```python
from build123d import *

# Parameters (mm, degrees)
F1_DEPTH = 150
F3_DEPTH = 200
F5_DEPTH = 100
F6_R     = 5
F7_R     = 5
F8_R     = 5
F9_R     = 5
F10_R    = 5
F11_R    = 5
F12_R    = 5


with BuildPart() as f1:
    # F0 (on Front) → F1 (new body)
    with BuildSketch(Plane.XZ):
        Polygon((2.699633, 10.554306), (13.111226, -10.555131), (91.699633, 13.444814), (91.699633, 51.205629), (2.699633, 51.205629), (-87.100367, 51.205629), (-87.100367, 12.852651), (-8.070518, -11.282105), align=None)
    extrude(amount=F1_DEPTH)

    # F2 (on face) → F3 (cut)
    with BuildSketch(Plane(origin=(0, 0, 0), x_dir=(-1, 0, 0), z_dir=(0, 1, 0))):
        Polygon((10.674811, -5.258827), (82.100367, 16.55367), (82.100367, 46.205629), (-86.699632, 46.205629), (-86.699632, 17.145834), (-15.715518, -4.531853), (-2.699633, 21.857769), align=None)
    extrude(amount=-F3_DEPTH, mode=Mode.SUBTRACT)

    # F4 (on face) → F5 (intersect)
    with BuildSketch(Plane.XY.offset(51.205629)):
        with BuildLine():
            Line((105.917034, -74.399856), (110.162811, -71.75914))
            ThreePointArc((110.162811, -71.75914), (-2.511346, -9.56452), (-114.475567, -73.028285))
            Line((-114.475567, -73.028285), (-110.200224, -75.620859))
            ThreePointArc((-110.200224, -75.620859), (-2.483098, -14.564441), (105.917034, -74.399856))
        make_face()
    extrude(amount=-F5_DEPTH, mode=Mode.INTERSECT)

    # F6
    f6_edges = [f1.edges().sort_by_distance(p)[0] for p in [
        (2.699633, -12.139598, 21.857769),
    ]]
    fillet(f6_edges, radius=F6_R)

    # F7
    f7_edges = [f1.edges().sort_by_distance(p)[0] for p in [
        (-8.070518, -12.216219, -11.282105),
    ]]
    fillet(f7_edges, radius=F7_R)

    # F8
    f8_edges = [f1.edges().sort_by_distance(p)[0] for p in [
        (13.111226, -12.92147, -10.555131),
    ]]
    fillet(f8_edges, radius=F8_R)

    # F9
    f9_edges = [f1.edges().sort_by_distance(p)[0] for p in [
        (-87.100367, -44.240648, 51.205629),
    ]]
    fillet(f9_edges, radius=F9_R)

    # F10
    f10_edges = [f1.edges().sort_by_distance(p)[0] for p in [
        (-87.100367, -44.240648, 12.852651),
    ]]
    fillet(f10_edges, radius=F10_R)

    # F11
    f11_edges = [f1.edges().sort_by_distance(p)[0] for p in [
        (91.699633, -52.049978, 51.205629),
    ]]
    fillet(f11_edges, radius=F11_R)

    # F12
    f12_edges = [f1.edges().sort_by_distance(p)[0] for p in [
        (91.699633, -52.049978, 13.444814),
    ]]
    fillet(f12_edges, radius=F12_R)


solid = f1.part
```
Can you work these out from the model? Positions are in its coordinate system, mm. A direction names the side the tool comes from. Give positions to 0.01 mm unless a question says otherwise; leave off trailing zeros. Order: outer loops, then holes, each group sorted by start corner. A loop starts at its lowest first (then second) coordinate and runs counter-clockwise, first axis right, second up. Notation, with made-up numbers: M 3,-10 L 24,-10 A7 ccw 24,-2 Z; hole C -13.5,-37.75 d4. An arc over 180 degrees is marked long. One line per item, written item: value.
1) I want a section at A-A, the plane z = 24.5. List the corners of the cut face in (x, y) for me.
Answer sheet:
outline: M -87.1,-47.57 A126.81 cw -82.1,-43.25 L -82.1,-36.87 A131.81 ccw -87.1,-40.91 Z; M 86.7,-50.52 A126.81 cw 91.7,-55.67 L 91.7,-48.43 A131.81 ccw 86.7,-43.66 Z
2) I want a section at D-D, the plane z = -2.5. List the corners of the cut face in (x, y) for me.
Answer sheet:
outline: M -36.83,-19.51 A126.81 cw -19.71,-15.84 L -19.71,-10.79 A131.81 ccw -36.83,-14.31 Z; M -9.31,-14.79 A126.81 cw -3.74,-14.58 L -3.74,-9.58 A131.81 ccw -9.31,-9.78 Z; M 9.14,-15.03 A126.81 cw 14.71,-15.64 L 14.71,-10.6 A131.81 ccw 9.14,-10.01 Z; M 22.37,-16.88 A126.81 cw 39.49,-21.46 L 39.49,-16.18 A131.81 ccw 22.37,-11.79 Z
3) I want a section at C-C, the plane y = -33. List the corners of the cut face in (x, z) for me.
Answer sheet:
outline: M -76.8,9.71 L -67.62,6.9 L -67.62,12.13 L -76.8,14.93 Z; M -76.8,46.21 L -67.62,46.21 L -67.62,51.21 L -76.8,51.21 Z; M 64.08,5.01 L 73.26,7.81 L 73.26,13.04 L 64.08,10.24 Z; M 64.08,46.21 L 73.26,46.21 L 73.26,51.21 L 64.08,51.21 Z
4) On a 3-axis mill with a long thin cutter (end or side, diameter ignored), from which of +Z, -Z, +X, -X, +Y, -Y can I reach the whole of each face in a straight line? I mean faces 5 (the face through (-6.167, -12.182, 3.88)), 6 (the face through (90.196, -49.748, 49.78)). Say none if no direction works.
Answer sheet:
face 5: +Y, -Y
face 6: +Z, +X, +Y, -Y
5) I want a section at B-B, the plane x = 24.5. List the corners of the cut face in (y, z) for me.
Answer sheet:
outline: M -17.31,-7.08 L -12.21,-7.08 L -12.21,-1.85 L -17.31,-1.85 Z; M -17.31,46.21 L -12.21,46.21 L -12.21,51.21 L -17.31,51.21 Z
6) For P1, Ø3, axis at y = -39.5, z = 35.5, coming from the +X side; P2, Ø2, axis at y = -24, z = 4.5, coming from the -X side; P3, Ø10, axis at y = -21.5, z = 4, coming from the +X side, each with a flat end and sliding along its axis, tell me the tip position at first contact or that it passes through.
Answer sheet:
P1: stops at x = -82.1
P2: stops at x = -62.65
P3: stops at x = 62.8
7) Please list where these lines run through material, in increasing order: line 1 along X through (y, z) = (-50.5, 19); line 2 along Z through (x, y) = (-68, -32); line 3 along Z through (x, y) = (-18.5, -14).
Answer sheet:
line 1: x = 86.7 to 91.7
line 2: z = 7.02 to 12.25, 46.21 to 51.21
line 3: z = -8.1 to -2.87, 46.21 to 51.21
8) We'd pull the mould along X, two halves only. Please class faces 1 (the face through (-87.1, -44, 32)), 2 (the face through (4.23, -9.7, 11.48)), 3 (the face through (-8.74, -12.35, -9.87)), 4 (the face through (8.9, -14.8, 51.206)): released by +X, released by -X, zero draft, split by the parting line, or undercut.
Answer sheet:
face 1: released by -X
face 2: split by the parting line
face 3: undercut
face 4: zero draft
